Part print with two shaded views. Sizes in mm from the minimum x, y, z corner. Round coordinates to 2 decimals unless told otherwise and drop trailing zeros. Loops run counter-clockwise (first coordinate to the right, second up) from the corner with the lowest first, then second, coordinate; pieces in that order, holes last. Notation, with made-up numbers: (86.5, 49) - (145.5, 49) arc R28 ccw to (145.5, 70) - close; hole circle Ø3 at (3.5, 64.5). An arc over 180 degrees is marked (long way). Put each result on its own line as item: value. Start each with the question number.
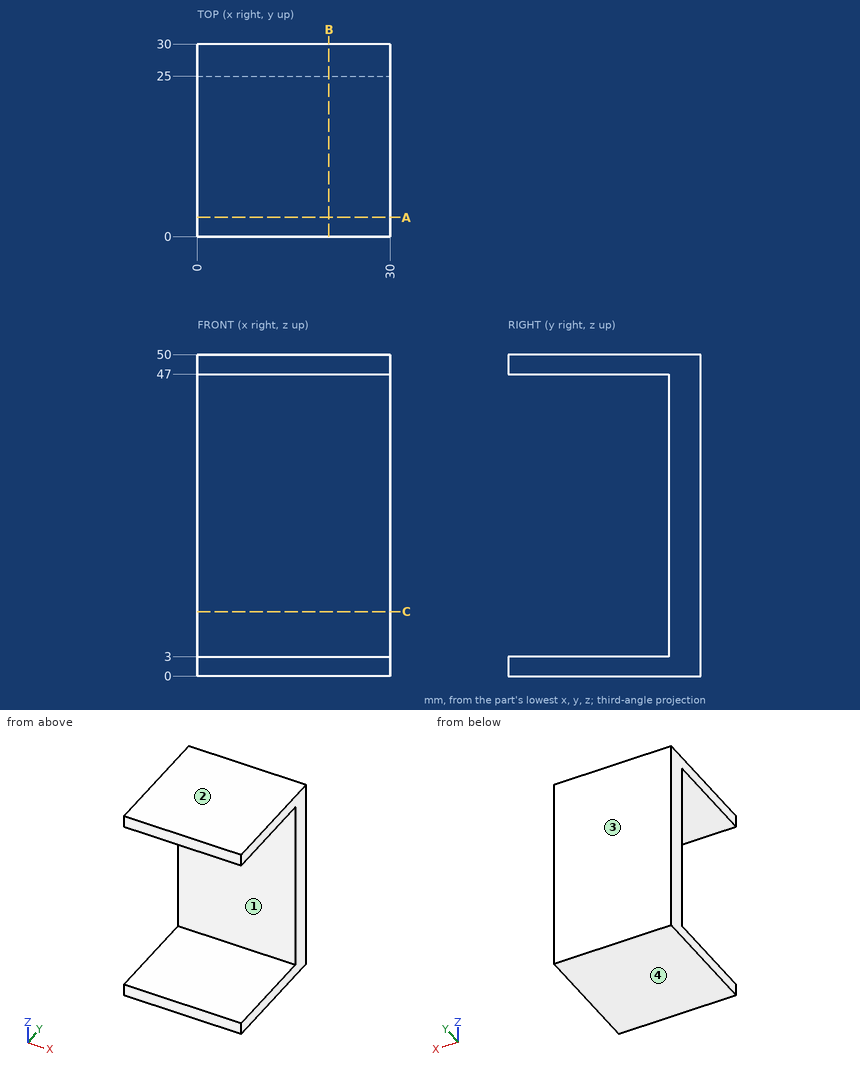
1) Slice it at B-B, the plane x = 20.5. Write the cut outline in (y, z).
2) Slice it at C-C, the plane z = 10. Write the cut outline in (x, y), and give its area (3 significant figures).
3) Drill centre lines: line 1 (Z direction, x = 2, y = 12); line 2 (Y direction, x = 27, z = 46.5). Where is each one in solid material? Low to high. Write a range as [from, to].
4) Pull direction Z, two halves, no side cores. Call the marked faces 1, 2, 3 and 4: pulls with the +Z half, pulls with the -Z half, needs draft (parallel to the pull), parting line crosses it, or undercut.
5) Drop a flat-ended pin along its axis: pin 1 Ø2 at (x, z) = (20, 43.5) entering from -Y. Give the stop position or say it passes through.
6) Slice it at A-A, the plane y = 3. Write the cut outline in (x, z), and give its area (3 significant figures).
Taken from the geometry:
1. outline: (0, 0) - (30, 0) - (30, 50) - (0, 50) - (0, 47) - (25, 47) - (25, 3) - (0, 3) - close
2. outline: (0, 25) - (30, 25) - (30, 30) - (0, 30) - close
2. area: 150 mm2
3. line 1: z = [0, 3], [47, 50]
3. line 2: y = [25, 30]
4. face 1: undercut
4. face 2: pulls with the +Z half
4. face 3: needs draft
4. face 4: pulls with the -Z half
5. pin 1: stops at y = 25
6. outline: (0, 0) - (30, 0) - (30, 3) - (0, 3) - close; (0, 47) - (30, 47) - (30, 50) - (0, 50) - close
6. area: 180 mm2
